Here's how the part is built. I have some questions about the finished solid (model axes, mm). A direction names the side the tool comes from. Round coordinates to 2 decimals unless told otherwise and drop trailing zeros. Write each loop counter-clockwise with the first axis right and the second up, starting at its lowest first coordinate (ties: lowest second). Pieces come first, ordered by that corner, then holes. Notation, with made-up numbers: (67.5, -7) -> (118.5, -7) arc R17 cw to (118.5, 11) -> close; hole circle Ø8 at (10.5, -6.75). An arc over 180 degrees is marked (long way). Put each result on its own line as item: value. Start each with the question number.
1. I need wall thicknesses on probe 1 along X at (y, z) = (-16.5, -214.5); probe 2 along Z at (x, y) = (95, -21); probe 3 along X at (y, z) = (-1.5, -11.5). Which ranges of each line are inside material? Lowest first, please. Write a range as from..to.
2. We'd pull the mould along X, two halves only. Please class faces 3 (the face through (-150, -15, -122)), 4 (the face through (144.297, -14.79, -7.014)), 5 (the face through (-151, -15, -125)), 6 (the face through (-150.493, -14.67, -225.996)): +X half, -X half, draft (parallel to the pull), parting line (faces both ways), or undercut.
3. For pin 1 (1.1 mm diameter, centred on x = 150.5, y = -16, fed in from -Z); pin 2 (0.8 mm diameter, centred on x = -150.5, z = -212, fed in from -Y), each with a flat end and sliding along its axis, tell me the tip position at first contact or that it passes through.
4. Which directions (+Z, -Z, +X, -X, +Y, -Y) give clear straight access to the entire face, cutting with the end or side of a thin tool? Please do faces 1 (the face through (2, -15, -1)), 2 (the face through (-145.012, -14.79, -6.315)).
5. Suppose I cut it at B-B (y = -7.75). Please give me the cut outline in (x, z).
6. Suppose I cut it at A-A (z = -16). Please give me the cut outline in (x, y).
7. Suppose I cut it at D-D (x = -108.5). Please give me the cut outline in (y, z).
8. Suppose I cut it at C-C (z = -174). Please give me the cut outline in (x, y), then the cut area to 3 significant figures.
```python
from build123d import *

# Parameters (mm, degrees)
LINEAR_AUSTRAGEN_D_NN1_DEPTH    = 30
SCHNITT_LINEAR_AUSTRAGEN1_DEPTH = 303
SKIZZE5_W                       = 6
SKIZZE5_H                       = 6
SCHNITT_LINEAR_AUSTRAGEN2_DEPTH = 303


with BuildPart() as part:
    # Skizze3 → Linear-Austragen-Dünn1 (new body)
    with BuildSketch(Plane.XZ):
        with BuildLine():
            Line((-151, -226), (-151, -151))
            Line((-151, -151), (-151, -21))
            ThreePointArc((-151, -21), (-144.849242405, -6.150757595), (-130, 0))
            Line((-130, 0), (130, 0))
            ThreePointArc((130, 0), (144.849242405, -6.150757595), (151, -21))
            Line((151, -21), (151, -151))
            Line((151, -151), (151, -226))
            Line((151, -226), (150, -226))
            Line((150, -226), (150, -151))
            Line((150, -151), (150, -21))
            ThreePointArc((150, -21), (144.142135624, -6.857864376), (130, -1))
            Line((130, -1), (-130, -1))
            ThreePointArc((-130, -1), (-144.142135624, -6.857864376), (-150, -21))
            Line((-150, -21), (-150, -151))
            Line((-150, -151), (-150, -226))
            Line((-150, -226), (-151, -226))
        make_face()
    extrude(amount=LINEAR_AUSTRAGEN_D_NN1_DEPTH)

    # Skizze4 → Schnitt-Linear austragen1 (cut, through all)
    with BuildSketch(Plane(origin=(151, 0, 0), x_dir=(0, 0, -1), z_dir=(1, 0, 0))):
        with BuildLine():
            Line((236.953367606, 0), (211, 0))
            ThreePointArc((211, 0), (226, -15), (211, -30))
            Line((211, -30), (236.953367606, -30))
            Line((236.953367606, -30), (236.953367606, 0))
        make_face()
    extrude(amount=-SCHNITT_LINEAR_AUSTRAGEN1_DEPTH, mode=Mode.SUBTRACT)

    # Skizze5 → Schnitt-Linear austragen2 (cut, through all)
    with BuildSketch(Plane(origin=(151, 0, 0), x_dir=(0, 0, -1), z_dir=(1, 0, 0))):
        with Locations((211, -15)):
            Rectangle(SKIZZE5_W, SKIZZE5_H)
    extrude(amount=-SCHNITT_LINEAR_AUSTRAGEN2_DEPTH, mode=Mode.SUBTRACT)


solid = part.part
```
Verdict:
1. probe 1: x = -151..-150, 150..151
1. probe 2: z = -1..0
1. probe 3: x = -148.73..-147.6, 147.6..148.73
2. face 3: undercut
2. face 4: undercut
2. face 5: -X half
2. face 6: draft
3. pin 1: stops at z = -225.99
3. pin 2: stops at y = -29.99
4. face 1: -Z, +Y, -Y
4. face 2: +Z, -X, +Y, -Y
5. outline: (-151, -224.13) -> (-150, -224.13) -> (-150, -21) arc R20 cw to (-130, -1) -> (130, -1) arc R20 cw to (150, -21) -> (150, -224.13) -> (151, -224.13) -> (151, -21) arc R21 ccw to (130, 0) -> (-130, 0) arc R21 ccw to (-151, -21) -> close
6. outline: (-150.4, -30) -> (-149.36, -30) -> (-149.36, 0) -> (-150.4, 0) -> close; (149.36, -30) -> (150.4, -30) -> (150.4, 0) -> (149.36, 0) -> close
7. outline: (-30, -1) -> (0, -1) -> (0, 0) -> (-30, 0) -> close
8. outline: (-151, -30) -> (-150, -30) -> (-150, 0) -> (-151, 0) -> close; (150, -30) -> (151, -30) -> (151, 0) -> (150, 0) -> close
8. area: 60.0 mm^2
